Design review of the part built by this model. Coordinates are the model's own, in mm. A direction names the side the tool comes from. Coordinates: 2 decimals unless noted, no trailing zeros. Return JSON: item names as keys, results as strings. Group by question number.
```python
from build123d import *

# Parameters (mm, degrees)
F0_W          = 50
F0_H          = 100
F1_DEPTH      = 50
F1_DEPTH_BACK = 50
F3_D          = 11
F3_DEPTH      = 12
F3_TIP        = 3.3047334047


with BuildPart() as f1:
    # F0 (on Top) → F1 (new body, two sides)
    with BuildSketch(Plane.XY) as f1_sk:
        Rectangle(F0_W, F0_H)
    extrude(amount=F1_DEPTH)
    extrude(f1_sk.sketch, amount=-F1_DEPTH_BACK)

    # F3
    with Locations(Plane(origin=(-25, 0, 0), x_dir=(0, -1, 0), z_dir=(-1, 0, 0))):
        with Locations((-40, 35), (30, 26), (3.0545412681, 0), (30, -30), (-40, -30)):
            Hole(F3_D / 2, depth=F3_DEPTH)
            with Locations((0, 0, -(F3_DEPTH + F3_TIP / 2))):  # 118° drill point
                Cone(0, F3_D / 2, F3_TIP, mode=Mode.SUBTRACT)


solid = f1.part
```
Item 1: For line 1 (Z direction, x = -16, y = 40); line 2 (Z direction, x = -16, y = -30); line 3 (Y direction, x = -17, z = -30), list the stretches that pass through material, from the lowest coordinate up.
Item 2: For pin 1 (9 mm diameter, centred on y = -30, z = -30, fed in from -X), flat-tipped, find the tip position at first contact; note if it passes through.
Item 3: The part is to be moulded in two halves that separate along Z. For faces 3 (the flat face through (0, 1, -50)), 4 (the flat face through (-25, -12, 1)), 5 (the cylindrical face through (-18.916, -35.495, 26.242)), 6 (the cylindrical face through (-18.916, 2.026, -2.107)), say which applies: pulls with the +Z half, pulls with the -Z half, needs draft (parallel to the pull), parting line crosses it, or undercut.
Item 4: Machinability: for faces 1 (the flat face through (0, -50, 1)), 2 (the cylindrical face through (-18.916, 34.505, -29.758)), which of the approach directions +Z, -Z, +X, -X, +Y, -Y give a long, thin tool a straight path to every point of the face, cutting with its end or side? Answer none if there is none.
Geometry check:
{
 "1": {"line 1": "-50 to -35.5, -24.5 to 29.5, 40.5 to 50", "line 2": "-50 to -35.5, -24.5 to 20.5, 31.5 to 50", "line 3": "-50 to -35.5, -24.5 to 34.5, 45.5 to 50"},
 "2": {"pin 1": "x = -12.4"},
 "3": {"face 3": "pulls with the -Z half", "face 4": "needs draft", "face 5": "undercut", "face 6": "undercut"},
 "4": {"face 1": "+Z, -Z, +X, -X, -Y", "face 2": "-X"}
}
